Check sheet for the modelled part. Datum: model origin and axes. Units: mm. A direction names the side the tool comes from. Round coordinates to 2 decimals unless told otherwise and drop trailing zeros. Order: outer loops, then holes, each group sorted by start corner. A loop starts at its lowest first (then second) coordinate and runs counter-clockwise, first axis right, second up. Notation, with made-up numbers: (52.5, 75) -> (67.5, 75) arc R36 ccw to (67.5, 113) -> close; hole circle Ø10 at (-10.75, -32.75). An arc over 180 degrees is marked (long way). Answer in a Markdown table with one row per item.
from build123d import *

# Parameters (mm, degrees)
CROQUIS1_W              = 100
CROQUIS1_H              = 100
PLACABASE_DEPTH         = 3
CROQUIS2_W              = 100
CROQUIS2_H              = 100
CROQUIS2_W_2            = 95.2
CROQUIS2_H_2            = 95.2
PAREDES_DEPTH           = 21
CROQUIS4_W              = 26.4
CROQUIS4_H              = 10.4
ALOJAMIENTOSMOTOR_DEPTH = 12.4
CROQUIS6_W              = 2.4
CROQUIS6_H              = 95.2
NERVIOSRIGIDEZ_DEPTH    = 9
CROQUIS7_W              = 95.2
CROQUIS7_H              = 6
BLOQUECUNA_DEPTH        = 10
CROQUIS8_W              = 44
CROQUIS8_H              = 4
TORRESENSORES_DEPTH     = 22
CROQUIS11_W             = 2.875664279
CROQUIS11_H             = 12.708105518
CROQUIS11_W_2           = 2.4
NERVIOSTORRE_DEPTH      = 22
CROQUIS12_R             = 4
POSTESPLACA_DEPTH       = 18


with BuildPart() as part:
    # Croquis1 → PlacaBase (new body)
    with BuildSketch(Plane(origin=(0, 0, 0), x_dir=(1, 0, 0), z_dir=(0, 1, 0))):
        with Locations((50, 50)):
            Rectangle(CROQUIS1_W, CROQUIS1_H)
    extrude(amount=PLACABASE_DEPTH)

    # Croquis2 → Paredes (add)
    with BuildSketch(Plane(origin=(0, 3, 0), x_dir=(1, 0, 0), z_dir=(0, 1, 0))):
        with Locations((50, 50)):
            Rectangle(CROQUIS2_W, CROQUIS2_H)
        with Locations((50, 50)):
            Rectangle(CROQUIS2_W_2, CROQUIS2_H_2, mode=Mode.SUBTRACT)
    extrude(amount=PAREDES_DEPTH)

    # Croquis4 → AlojamientosMotor (cut)
    with BuildSketch(Plane(origin=(0, 7.3, 0), x_dir=(1, 0, 0), z_dir=(0, 1, 0))):
        with Locations((27.2, 72)):
            Rectangle(CROQUIS4_W, CROQUIS4_H)
        with Locations((72.8, 72)):
            Rectangle(CROQUIS4_W, CROQUIS4_H)
    extrude(amount=-ALOJAMIENTOSMOTOR_DEPTH, mode=Mode.SUBTRACT)

    # Croquis6 → NerviosRigidez (add)
    with BuildSketch(Plane(origin=(0, 3, 0), x_dir=(1, 0, 0), z_dir=(0, 1, 0))):
        with Locations((18.2, 50)):
            Rectangle(CROQUIS6_W, CROQUIS6_H)
        with Locations((81.8, 50)):
            Rectangle(CROQUIS6_W, CROQUIS6_H)
    extrude(amount=NERVIOSRIGIDEZ_DEPTH)

    # Croquis7 → BloqueCuna (add)
    with BuildSketch(Plane(origin=(0, 3, 0), x_dir=(1, 0, 0), z_dir=(0, 1, 0))):
        with Locations((50, 5.4)):
            Rectangle(CROQUIS7_W, CROQUIS7_H)
    extrude(amount=BLOQUECUNA_DEPTH)

    # Croquis8 → TorreSensores (add)
    with BuildSketch(Plane(origin=(0, 3, 0), x_dir=(1, 0, 0), z_dir=(0, 1, 0))):
        with Locations((50, 10.4)):
            Rectangle(CROQUIS8_W, CROQUIS8_H)
    extrude(amount=TORRESENSORES_DEPTH)

    # Croquis11 → NerviosTorre (add)
    with BuildSketch(Plane(origin=(0, 3, 0), x_dir=(1, 0, 0), z_dir=(0, 1, 0))):
        with Locations((29.43783214, 18.754052759)):
            Rectangle(CROQUIS11_W, CROQUIS11_H)
        with Locations((70.8, 18.754052759)):
            Rectangle(CROQUIS11_W_2, CROQUIS11_H)
    extrude(amount=NERVIOSTORRE_DEPTH)

    # Croquis12 → PostesPlaca (add)
    with BuildSketch(Plane(origin=(0, 3, 0), x_dir=(1, 0, 0), z_dir=(0, 1, 0))):
        with Locations(Location((18, 26, 0), (0, 0, 104.477512186))):
            Circle(CROQUIS12_R)
        with Locations(Location((82, 26, 0), (0, 0, 75.522487814))):
            Circle(CROQUIS12_R)
        with Locations(Location((18, 58, 0), (0, 0, 104.477512186))):
            Circle(CROQUIS12_R)
        with Locations(Location((82, 58, 0), (0, 0, 75.522487814))):
            Circle(CROQUIS12_R)
    extrude(amount=POSTESPLACA_DEPTH)


solid = part.part
Item 1: Depth check by flat-ended pin: P1, Ø12, axis at x = 20.5, z = -26.5, coming from the +Y side; P2, Ø1.2, axis at x = 81.5, z = -12.5, coming from the +Y side; P3, Ø7.5, axis at x = 94, z = -35.5, coming from the +Y side. Enter the tip coordinate at first touch or a pass-through.
Result sheet:
| item | result |
|---|---|
| P1 | stops at y = 21 |
| P2 | stops at y = 12 |
| P3 | stops at y = 24 |
Item 2: Cross-section at C-C (z = -11). Record the boundary of the cut face in (x, y).
Result sheet:
| item | result |
|---|---|
| outline | (0, 0) -> (100, 0) -> (100, 24) -> (97.6, 24) -> (97.6, 3) -> (83, 3) -> (83, 12) -> (80.6, 12) -> (80.6, 3) -> (72, 3) -> (72, 25) -> (28, 25) -> (28, 3) -> (19.4, 3) -> (19.4, 12) -> (17, 12) -> (17, 3) -> (2.4, 3) -> (2.4, 24) -> (0, 24) -> close |
Item 3: Mould release check, pull along Z, two halves, no side actions. Record for faces 4 (the flat face through (49, 18, -2.4)), 5 (the flat face through (50, 19, -8.4)), 6 (the flat face through (46, 24, -2)): pulls with the +Z half, pulls with the -Z half, needs draft (parallel to the pull), parting line crosses it, or undercut.
Result sheet:
| item | result |
|---|---|
| face 4 | undercut |
| face 5 | undercut |
| face 6 | needs draft |
Item 4: Cross-section at D-D (x = 46). Record the boundary of the cut face in (y, z).
Result sheet:
| item | result |
|---|---|
| outline | (0, -100) -> (24, -100) -> (24, -97.6) -> (3, -97.6) -> (3, -12.4) -> (25, -12.4) -> (25, -8.4) -> (13, -8.4) -> (13, -2.4) -> (24, -2.4) -> (24, 0) -> (0, 0) -> close |
Item 5: Scan lines: line 1 (Z direction, x = 48, y = 14.75); line 2 (X direction, y = 8.5, z = -88.5); line 3 (Z direction, x = 75, y = 18.5). Record each from-to range of solid material in increasing order. Write a range as [from, to].
Result sheet:
| item | result |
|---|---|
| line 1 | z = [-100, -97.6], [-12.4, -8.4], [-2.4, 0] |
| line 2 | x = [0, 2.4], [17, 19.4], [80.6, 83], [97.6, 100] |
| line 3 | z = [-100, -97.6], [-2.4, 0] |
Item 6: Cross-section at B-B (x = 67). Record the boundary of the cut face in (y, z), and give its area (3 significant figures).
Result sheet:
| item | result |
|---|---|
| outline | (0, -100) -> (24, -100) -> (24, -97.6) -> (3, -97.6) -> (3, -77.2) -> (0, -77.2) -> close; (0, -66.8) -> (3, -66.8) -> (3, -12.4) -> (25, -12.4) -> (25, -8.4) -> (13, -8.4) -> (13, -2.4) -> (24, -2.4) -> (24, 0) -> (0, 0) -> close |
| area | 518 mm^2 |
Item 7: Cross-section at A-A (y = 16.5). Record the boundary of the cut face in (x, z), and give its area (3 significant figures).
Result sheet:
| item | result |
|---|---|
| outline | (0, -100) -> (100, -100) -> (100, 0) -> (0, 0) -> close; circle Ø8 at (18, -58); circle Ø8 at (18, -26); (28, -25.11) -> (30.88, -25.11) -> (30.88, -12.4) -> (69.6, -12.4) -> (69.6, -25.11) -> (72, -25.11) -> (72, -8.4) -> (28, -8.4) -> close; circle Ø8 at (82, -58); circle Ø8 at (82, -26); hole (2.4, -97.6) -> (97.6, -97.6) -> (97.6, -2.4) -> (2.4, -2.4) -> close |
| area | 1,380 mm^2 |
Item 8: Set-up check for faces 1 (the flat face through (100, 12, -49)), 2 (the flat face through (40.4, 2, -72)), 3 (the flat face through (49, 13, -97.6)): record each of +Z, -Z, +X, -X, +Y, -Y from which the full face is reachable in a straight line by a thin tool's end or side.
Result sheet:
| item | result |
|---|---|
| face 1 | +Z, -Z, +X, +Y, -Y |
| face 2 | +Y, -Y |
| face 3 | +Y |
